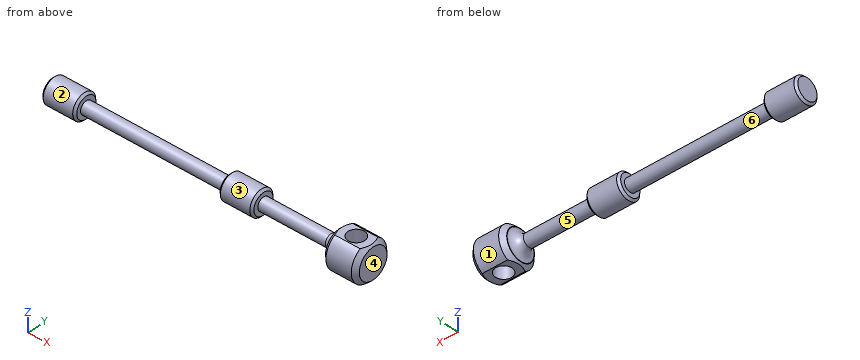
from build123d import *

# Parameters (mm, degrees)
SKETCH1_R           = 1.5
BOSS_EXTRUDE1_DEPTH = 38
SKETCH2_R           = 3
BOSS_EXTRUDE2_DEPTH = 8
BOSS_EXTRUDE3_START = -42
SKETCH2_2_R         = 3
BOSS_EXTRUDE3_DEPTH = 8
CHAMFER1_SIZE       = 0.5
SKETCH3_R           = 4.617370453
BOSS_EXTRUDE4_DEPTH = 8
CUT_EXTRUDE1_DEPTH  = 8
SKETCH5_R           = 2
CUT_EXTRUDE2_DEPTH  = 40.1065226
CHAMFER2_SIZE       = 1
FILLET1_R           = 2


with BuildPart() as part:
    # Sketch1 → Boss-Extrude1 (new, symmetric)
    with BuildSketch(Plane(origin=(0, 0, 0), x_dir=(0, 0, -1), z_dir=(1, 0, 0))):
        Circle(SKETCH1_R)
    extrude(amount=BOSS_EXTRUDE1_DEPTH, both=True)

    # Sketch2 → Boss-Extrude2 (add)
    with BuildSketch(Plane.ZY.offset(38)):
        Circle(SKETCH2_R)
    extrude(amount=-BOSS_EXTRUDE2_DEPTH)

    # Sketch2<2> → Boss-Extrude3 (add)
    with BuildSketch(Plane.ZY.offset(38).offset(BOSS_EXTRUDE3_START)):
        Circle(SKETCH2_2_R)
    extrude(amount=-BOSS_EXTRUDE3_DEPTH)

    # Chamfer1
    chamfer1_edges = [part.edges().sort_by_distance(p)[0] for p in [
        (12, 0, -3),
        (4, 0, -3),
        (-30, 0, -3),
        (-38, 0, -3),
    ]]
    chamfer(chamfer1_edges, length=CHAMFER1_SIZE)

    # Sketch3 → Boss-Extrude4 (add)
    with BuildSketch(Plane(origin=(38, 0, 0), x_dir=(0, 0, -1), z_dir=(1, 0, 0))):
        Circle(SKETCH3_R)
    extrude(amount=-BOSS_EXTRUDE4_DEPTH)

    # Sketch4 → Cut-Extrude1 (cut)
    with BuildSketch(Plane(origin=(38, 0, 0), x_dir=(0, 0, -1), z_dir=(1, 0, 0))):
        with BuildLine():
            Line((-4, 2.306536342), (-4, -2.306536342))
            ThreePointArc((-4, -2.306536342), (-4.617370453, 0), (-4, 2.306536342))
        make_face()
        with BuildLine():
            Line((4, 2.306536342), (4, -2.306536342))
            ThreePointArc((4, -2.306536342), (4.617370453, 0), (4, 2.306536342))
        make_face()
    extrude(amount=-CUT_EXTRUDE1_DEPTH, mode=Mode.SUBTRACT)

    # Sketch5 → Cut-Extrude2 (cut, through all)
    with BuildSketch(Plane.XY.offset(4)):
        with Locations((34, 0)):
            Circle(SKETCH5_R)
    extrude(amount=-CUT_EXTRUDE2_DEPTH, mode=Mode.SUBTRACT)

    # Chamfer2
    # the kernel refuses this chamfer: 1 mm, written as the material it takes off along each edge
    with BuildSketch(Plane(origin=(30, 0, 0), x_dir=(0, -0.03428839370133285, -0.9994119801450163), z_dir=(0, -0.9994119801450163, 0.03428839370133285))) as chamfer2_piece_1:
        Polygon((4.617370453 - CHAMFER2_SIZE, 0), (4.617370453, CHAMFER2_SIZE), (4.617370453, 0), align=None)
    revolve(axis=Axis((30, 0, 0), (1, 0, 0)), revolution_arc=183.929930813, mode=Mode.SUBTRACT)
    with BuildSketch(Plane(origin=(38, 0, 0), x_dir=(0, -0.0342883937013343, -0.9994119801450161), z_dir=(0, -0.9994119801450161, 0.0342883937013343))) as chamfer2_piece_2:
        Polygon((4.617370453, -CHAMFER2_SIZE), (4.617370453 - CHAMFER2_SIZE, 0), (4.617370453, 0), align=None)
    revolve(axis=Axis((38, 0, 0), (1, 0, 0)), revolution_arc=183.929930813, mode=Mode.SUBTRACT)
    with BuildSketch(Plane(origin=(38, 0, 0), x_dir=(0, 0.03428839370133442, 0.9994119801450161), z_dir=(0, 0.9994119801450161, -0.03428839370133442))) as chamfer2_piece_3:
        Polygon((4.617370453, -CHAMFER2_SIZE), (4.617370453 - CHAMFER2_SIZE, 0), (4.617370453, 0), align=None)
    revolve(axis=Axis((38, 0, 0), (1, 0, 0)), revolution_arc=183.929930813, mode=Mode.SUBTRACT)
    with BuildSketch(Plane(origin=(30, 0, 0), x_dir=(0, 0.034288393701332645, 0.9994119801450163), z_dir=(0, 0.9994119801450163, -0.034288393701332645))) as chamfer2_piece_4:
        Polygon((4.617370453 - CHAMFER2_SIZE, 0), (4.617370453, CHAMFER2_SIZE), (4.617370453, 0), align=None)
    revolve(axis=Axis((30, 0, 0), (1, 0, 0)), revolution_arc=183.929930813, mode=Mode.SUBTRACT)

    # Fillet1
    fillet1_edges = [part.edges().sort_by_distance(p)[0] for p in [
        (30, 0, 1.5),
    ]]
    fillet(fillet1_edges, radius=FILLET1_R)


solid = part.part
Geometry check sheet. Reference: the model listing, model coordinates, mm. Face numbers are marked on the shaded views. A direction names the side the tool comes from. Give positions to 0.01 mm unless a question says otherwise; leave off trailing zeros. Write each loop counter-clockwise with the first axis right and the second up, starting at its lowest first coordinate (ties: lowest second). Pieces come first, ordered by that corner, then holes. Notation, with made-up numbers: (-29.75, 35) - (19.25, 35) arc R28 ccw to (19.25, 53) - close; hole circle Ø10 at (61, 73.5). An arc over 180 degrees is marked (long way). Put each result on its own line as item: value.
1. Thickness scan on line 1 (X direction, y = 1.5, z = -2.25); line 2 (Y direction, x = 34, z = -0.25); line 3 (Y direction, x = 15, z = 0). Record the ranges inside material, lowest first.
Ans:
line 1: x = -37.8 to -30.2, 4.2 to 11.8, 29.83 to 32.68, 35.32 to 38
line 2: y = -4.61 to -2, 2 to 4.61
line 3: y = -1.5 to 1.5
2. Go/stop test with flat-tipped pins: pin 1 (4 mm diameter, centred on x = -6.5, y = 0.5, fed in from -Z); pin 2 (4 mm diameter, centred on x = 3, z = -3, fed in from +Y); pin 3 (5 mm diameter, centred on x = 13.5, y = -1, fed in from -Z); pin 4 (1 mm diameter, centred on x = -18.5, z = -2.5, fed in from +Y). Record where each tip stops, or that it passes through.
Ans:
pin 1: stops at z = -1.5
pin 2: stops at y = 2.49
pin 3: stops at z = -3
pin 4: passes through
3. Set-up check for the marked faces 1 and 2: record each of +Z, -Z, +X, -X, +Y, -Y from which the full face is reachable in a straight line by a thin tool's end or side.
Ans:
face 1: +X, -X, +Y
face 2: -X
4. Sectioned sample at C-C, the plane x = -32. Enter the section's corners in (y, z), plus the area to 3 significant figures.
Ans:
outline: circle Ø6 at (0, 0)
area: 28.3 mm²
5. Sectioned sample at A-A, the plane x = 34. Enter the section's corners in (y, z).
Ans:
outline: (-2.31, -4) - (-2, -4) - (-2, 4) - (-2.31, 4) arc R4.62 ccw to start; (2, -4) - (2.31, -4) arc R4.62 ccw to (2.31, 4) - (2, 4) - close
6. Sectioned sample at B-B, the plane x = -22.5. Enter the section's corners in (y, z), plus the area to 3 significant figures.
Ans:
outline: circle Ø3 at (0, 0)
area: 7.07 mm²
7. Draft check along X on the marked faces 3, 4, 5 and 6. Enter one of: +X half, -X half, draft (parallel to the pull), parting line (faces both ways), or undercut.
Ans:
face 3: draft
face 4: +X half
face 5: undercut
face 6: undercut
